from build123d import *

# Parameters (mm, degrees)
SKETCH1_W           = 152.4
SKETCH1_H           = 12.7
BOSS_EXTRUDE1_DEPTH = 25.4
BOSS_EXTRUDE2_DEPTH = 25.4
FILLET2_R           = 12.7


with BuildPart() as part:
    # Sketch1 → Boss-Extrude1 (new body)
    with BuildSketch(Plane(origin=(0, 129.522150418, 0), x_dir=(1, 0, 0), z_dir=(0, 1, 0))):
        with Locations((43.851863223, -12.926286206)):
            Rectangle(SKETCH1_W, SKETCH1_H)
    extrude(amount=-BOSS_EXTRUDE1_DEPTH)

    # Sketch2 → Boss-Extrude2 (add)
    with BuildSketch(Plane(origin=(0, 129.522150418, 0), x_dir=(1, 0, 0), z_dir=(0, 1, 0))):
        Polygon((-32.348136777, -6.576286206), (-32.348136777, 9.752049173), (-7.268775287, -6.576286206), (10.057684935, 9.752049173), (27.370150986, -6.576286206), (41.790569064, 9.752049173), (60.472332517, -6.576286206), (78.078963356, 9.752049173), (90.818027749, -6.576286206), (117.678669506, 9.752049173), (120.051863223, -6.576286206), (120.051863223, -10.496577103), (-32.348136777, -10.496577103), align=None)
    extrude(amount=-BOSS_EXTRUDE2_DEPTH)

    # Fillet2
    # the kernel refuses this fillet: 12.7 mm, written as the material it takes off along each edge
    with BuildSketch(Plane(origin=(-58.955745883, 129.522150418, -27.075375577), x_dir=(0, -1, 0), z_dir=(0.8380349324532734, 0, 0.5456165796491502))) as fillet2_piece_1_section:
        with BuildLine():
            CenterArc((FILLET2_R, -FILLET2_R), FILLET2_R, 90, 90)
            Line((0, -FILLET2_R), (0, 0))
            Line((0, 0), (FILLET2_R, 0))
        make_face()
    fillet2_piece_1 = extrude(amount=93.426391514, mode=Mode.PRIVATE)
    fillet2_piece_1 = split(fillet2_piece_1, bisect_by=Plane(origin=(-14.62978652, 126.629320204, 13.5132519), z_dir=(-0.6858340421816573, 0, -0.7277579725326055)), keep=Keep.TOP, mode=Mode.PRIVATE)
    add(fillet2_piece_1, mode=Mode.SUBTRACT)
    with BuildSketch(Plane(origin=(-30.375090914, 129.522150418, 28.351517045), x_dir=(0, -1, 0), z_dir=(0.7277579725326055, 0, -0.6858340421816573))) as fillet2_piece_2_section:
        with BuildLine():
            CenterArc((FILLET2_R, -FILLET2_R), FILLET2_R, 90, 90)
            Line((0, -FILLET2_R), (0, 0))
            Line((0, 0), (FILLET2_R, 0))
        make_face()
    fillet2_piece_2 = extrude(amount=87.307997817, mode=Mode.PRIVATE)
    fillet2_piece_2 = split(fillet2_piece_2, bisect_by=Plane(origin=(0.600633599, 126.627355979, 11.699795733), z_dir=(0.5456165796491502, 0, -0.8380349324532734)), keep=Keep.TOP, mode=Mode.PRIVATE)
    add(fillet2_piece_2, mode=Mode.SUBTRACT)
    with BuildSketch(Plane(origin=(113.112040831, 129.522150418, -41.171921906), x_dir=(0, -1, 0), z_dir=(0.14383082440379222, 0, 0.9896022907973312))) as fillet2_piece_3:
        with BuildLine():
            CenterArc((FILLET2_R, -FILLET2_R), FILLET2_R, 90, 90)
            Line((0, -FILLET2_R), (0, 0))
            Line((0, 0), (FILLET2_R, 0))
        make_face()
    extrude(amount=79.999896505, mode=Mode.SUBTRACT)
    with BuildSketch(Plane(origin=(63.687529345, 129.522150418, 23.068664941), x_dir=(0, -1, 0), z_dir=(0.8545038867379449, 0, -0.5194449995425362))) as fillet2_piece_4_section:
        with BuildLine():
            CenterArc((FILLET2_R, -FILLET2_R), FILLET2_R, 90, 90)
            Line((0, -FILLET2_R), (0, 0))
            Line((0, 0), (FILLET2_R, 0))
        make_face()
    fillet2_piece_4 = extrude(amount=94.934194945, mode=Mode.PRIVATE)
    fillet2_piece_4 = split(fillet2_piece_4, bisect_by=Plane(origin=(94.83379058, 126.638697733, 11.723502696), z_dir=(0.7884329224399922, 0, -0.61512074165381)), keep=Keep.TOP, mode=Mode.PRIVATE)
    add(fillet2_piece_4, mode=Mode.SUBTRACT)
    with BuildSketch(Plane(origin=(58.548879808, 129.522150418, -34.784794461), x_dir=(0, -1, 0), z_dir=(0.61512074165381, 0, 0.7884329224399922))) as fillet2_piece_5_section:
        with BuildLine():
            CenterArc((FILLET2_R, -FILLET2_R), FILLET2_R, 90, 90)
            Line((0, -FILLET2_R), (0, 0))
            Line((0, 0), (FILLET2_R, 0))
        make_face()
    fillet2_piece_5 = extrude(amount=84.209859919, mode=Mode.PRIVATE)
    fillet2_piece_5 = split(fillet2_piece_5, bisect_by=Plane(origin=(85.773780616, 126.63700346, 9.642637325), z_dir=(-0.5194449995425363, 0, -0.8545038867379451)), keep=Keep.TOP, mode=Mode.PRIVATE)
    add(fillet2_piece_5, mode=Mode.SUBTRACT)
    with BuildSketch(Plane(origin=(17.884716168, 129.522150418, -30.646371305), x_dir=(0, -1, 0), z_dir=(0.7529402486677585, 0, 0.6580888860451405))) as fillet2_piece_6_section:
        with BuildLine():
            CenterArc((FILLET2_R, -FILLET2_R), FILLET2_R, 90, 90)
            Line((0, -FILLET2_R), (0, 0))
            Line((0, 0), (FILLET2_R, 0))
        make_face()
    fillet2_piece_6 = extrude(amount=88.311747661, mode=Mode.PRIVATE)
    fillet2_piece_6 = split(fillet2_piece_6, bisect_by=Plane(origin=(56.205808832, 126.638654996, 10.533047171), z_dir=(-0.6799885276956249, 0, -0.7332227507397301)), keep=Keep.TOP, mode=Mode.PRIVATE)
    add(fillet2_piece_6, mode=Mode.SUBTRACT)
    with BuildSketch(Plane(origin=(-58.955745883, 129.522150418, -27.075375577), x_dir=(0, -1, 0), z_dir=(0.8380349324532734, 0, 0.5456165796491502))) as fillet2_piece_7a_section:
        with BuildLine():
            CenterArc((FILLET2_R, -FILLET2_R), FILLET2_R, 90, 90)
            Line((0, -FILLET2_R), (0, 0))
            Line((0, 0), (FILLET2_R, 0))
        make_face()
    fillet2_piece_7a = extrude(amount=93.426391514, mode=Mode.PRIVATE)
    fillet2_piece_7a = split(fillet2_piece_7a, bisect_by=Plane(origin=(-6.679987246, 126.680031692, 6.021416459), z_dir=(0.6858340421816573, 0, 0.7277579725326055)), keep=Keep.TOP, mode=Mode.PRIVATE)
    with BuildSketch(Plane(origin=(-30.375090914, 129.522150418, 28.351517045), x_dir=(0, -1, 0), z_dir=(0.7277579725326055, 0, -0.6858340421816573))) as fillet2_piece_7b_section:
        with BuildLine():
            CenterArc((FILLET2_R, -FILLET2_R), FILLET2_R, 90, 90)
            Line((0, -FILLET2_R), (0, 0))
            Line((0, 0), (FILLET2_R, 0))
        make_face()
    fillet2_piece_7b = extrude(amount=87.307997817, mode=Mode.PRIVATE)
    fillet2_piece_7b = split(fillet2_piece_7b, bisect_by=Plane(origin=(-7.946782213, 126.680031692, 6.134858521), z_dir=(-0.5456165796491502, 0, 0.8380349324532734)), keep=Keep.TOP, mode=Mode.PRIVATE)
    fillet2_piece_7 = fillet2_piece_7a & fillet2_piece_7b
    add(fillet2_piece_7, mode=Mode.SUBTRACT)
    with BuildSketch(Plane(origin=(58.548879808, 129.522150418, -34.784794461), x_dir=(0, -1, 0), z_dir=(0.61512074165381, 0, 0.7884329224399922))) as fillet2_piece_8a_section:
        with BuildLine():
            CenterArc((FILLET2_R, -FILLET2_R), FILLET2_R, 90, 90)
            Line((0, -FILLET2_R), (0, 0))
            Line((0, 0), (FILLET2_R, 0))
        make_face()
    fillet2_piece_8a = extrude(amount=84.209859919, mode=Mode.PRIVATE)
    fillet2_piece_8a = split(fillet2_piece_8a, bisect_by=Plane(origin=(89.912348573, 126.663062173, 7.126840189), z_dir=(0.5194449995425363, 0, 0.8545038867379451)), keep=Keep.TOP, mode=Mode.PRIVATE)
    with BuildSketch(Plane(origin=(63.687529345, 129.522150418, 23.068664941), x_dir=(0, -1, 0), z_dir=(0.8545038867379449, 0, -0.5194449995425362))) as fillet2_piece_8b_section:
        with BuildLine():
            CenterArc((FILLET2_R, -FILLET2_R), FILLET2_R, 90, 90)
            Line((0, -FILLET2_R), (0, 0))
            Line((0, 0), (FILLET2_R, 0))
        make_face()
    fillet2_piece_8b = extrude(amount=94.934194945, mode=Mode.PRIVATE)
    fillet2_piece_8b = split(fillet2_piece_8b, bisect_by=Plane(origin=(91.469987388, 126.663062173, 7.4119375), z_dir=(-0.7884329224399922, 0, 0.61512074165381)), keep=Keep.TOP, mode=Mode.PRIVATE)
    fillet2_piece_8 = fillet2_piece_8a & fillet2_piece_8b
    add(fillet2_piece_8, mode=Mode.SUBTRACT)


solid = part.part
Source: CAD feature listing. Evaluate the final solid. Frame: model axes, mm. A direction names the side the tool comes from. Coordinates: 2 decimals unless noted, no trailing zeros. Order: outer loops, then holes, each group sorted by start corner. A loop starts at its lowest first (then second) coordinate and runs counter-clockwise, first axis right, second up. Notation, with made-up numbers: M 46.25,-2 L 60.25,-2 A15 cw 60.25,27 Z; hole C 22,-10 d2. An arc over 180 degrees is marked long. Write each question's results on one line, items separated by ' | '. Start each with the question number.
Item 1: Cut plane B-B (z = 4). Count the separate pieces of the cut face and the enclosed holes in it, and give its area (3 significant figures).
Item 2: Line query: probe 1 along X at (y, z) = (118, 0.25); probe 2 along X at (y, z) = (114, -8); probe 3 along X at (y, z) = (125.5, -5). Output: solid intervals per line, ascending.
Item 3: Cut plane A-A (y = 125.75). Return loops of the section in (x, z), and give its area (3 significant figures).
Item 4: Set-up query: faces 1 (the face through (51.001, 110.561, -1.702)), 2 (the face through (43, 117, 19.276)), 3 (the face through (3.74, 125.703, 1.178)). Return all of +Z, -Z, +X, -X, +Y, -Y with unobstructed straight access to the full face (end or side cutting, diameter ignored); none if empty.
Item 5: Cut plane C-C (x = 29.5). Return loops of the section in (y, z).
Item 6: Cut plane D-D (y = 114.25). Return loops of the section in (x, z), and give its area (3 significant figures).
Item 7: Draft query along X for faces 4 (the face through (120.052, 114, 13)), 5 (the face through (103, 129.522, 17)), 6 (the face through (102.22, 125.7, 3.88)), 7 (the face through (-32.348, 117, 5)). Return one class per face: pulls with the +X half, pulls with the -X half, needs draft (parallel to the pull), parting line crosses it, or undercut.
Item 8: First-contact query: pin 1 Ø2 at (y, z) = (125, -3.5) entering from +X; pin 2 Ø1 at (y, z) = (117, 5.5) entering from +X. Flat tips, straight axial feed; report the tip coordinate or a pass-through.
Checked values:
1) separate pieces: 5 | enclosed holes: 0 | area: 2,950 mm2
2) probe 1: x = -32.35 to -17.09, -0.48 to 20.66, 32.96 to 53.15, 67.29 to 85.81, 101.33 to 119.08 | probe 2: x = -32.35 to -29.66, 8.2 to 11.92, 40.24 to 43.8, 76.19 to 79.45, 114.8 to 117.93 | probe 3: x = -32.35 to -31.33, 10.01 to 15.1, 37.59 to 42.02, 72.95 to 77.44
3) outline: M -32.35,-5.38 L -6.85,11.22 L 12.73,-7.23 L 27.37,6.58 L 39.36,-7 L 57.77,9.08 L 75.38,-7.25 L 89.93,11.41 L 114.85,-3.74 L 118.19,19.28 L -32.35,19.28 Z | area: 2,610 mm2
4) face 1: -Z, +Y, -Y | face 2: +Z, +X, -X, +Y, -Y | face 3: -Z, +Y
5) outline: M 104.12,4.16 L 129.52,4.16 L 129.52,19.28 L 104.12,19.28 Z
6) outline: M -32.35,-9.75 L -7.27,6.58 L 10.06,-9.75 L 27.37,6.58 L 41.79,-9.75 L 60.47,6.58 L 78.08,-9.75 L 90.82,6.58 L 117.68,-9.75 L 120.05,6.58 L 120.05,19.28 L -32.35,19.28 Z | area: 3,180 mm2
7) face 4: pulls with the +X half | face 5: needs draft | face 6: undercut | face 7: pulls with the -X half
8) pin 1: stops at x = 116.36 | pin 2: stops at x = 119.97
